Autodesk Inventor part; units mm, degrees
ref_plane "Work Plane3" through (0, 0, 2) normal (0, 0, 1) x (1, 0, 0)
ref_plane "Work Plane4" through (0, 0, -21) normal (0, 0, 1) x (1, 0, 0)
ref_plane "YZ Plane" through (0, 0, 0) normal (1, 0, 0) x (0, 1, 0)
sketch "Sketch1" plane through (0, 0, 0) normal (0, 1, 0) x (-1, 0, 0)
  line L0 (0, 0) -> (21, 0)
  circle A0 centre (5.5, 3.75) radius 1.5
  line L1 (29, 8) -> (-8, 8)
  line L2 (10.5, 8) -> (10.5, 0) construction
  line L3 (0, -21) -> (-8, -21)
  line L4 (29, 2) -> (72.5, 2)
  line L5 (72.5, 2) -> (72.5, 8)
  line L6 (72.5, 8) -> (29, 8)
  line L7 (29, 8) -> (29, 2)
  line L8 (21, 0) -> (21, 8)
  line L9 (0, 0) -> (0, 8)
  circle A1 centre (15.5, 3.75) radius 2.5
  line L10 (0, 0) -> (0, -21)
  line L11 (-8, -21) -> (-8, 8)
  line L12 (21, -21) -> (21, 0)
  line L13 (29, -21) -> (29, 2)
  line L14 (21, -21) -> (29, -21)
  circle A2 centre (-4, -10.5) radius 2.5
  circle A3 centre (25, -10.5) radius 1.5
  point P0 (29, 8)
  point P1 (21, 8)
  point P2 (-4, -21)
  dimension "d1" = 21
  dimension "d15" = 3.75
  dimension "d16" = 5
  dimension "d51" = 6
  dimension "d148" = 5
  dimension "d149" = 3.75
  dimension "d150" = 5
  dimension "d151" = 3
  dimension "d152" = 8
  dimension "d154" = 37
  dimension "d155" = 10.5
  dimension "d158" = 21
  dimension "d160" = 8
  dimension "d162" = 8
  dimension "d164" = 21
  dimension "d165" = 29
  dimension "d166" = 29
  dimension "d169" = 62
  dimension "d170" = 4
  dimension "d171" = 5
  dimension "d172" = 10.5
  dimension "d173" = 4
  dimension "d174" = 3
  dimension "d175" = 10.5
extrude "Extrusion1" add sketch "Sketch1" along normal mid plane 14 contours L9 L1 L8 L0 | L10 L3 L11 L1 L9 | L8 L1 L7 L13 L14 L12
extrude "Extrusion2" add sketch "Sketch1" along normal mid plane 25 contours L6 L5 L4 L7
fillet "Fillet4" radius 8 3 edges at (-72.5, 12.5, 5) (-72.5, -12.5, 5) (8, 0, 8)
ref_plane "Work Plane3" through (0, 0, 2) normal (0, 0, 1) x (1, 0, 0)
sketch "Sketch5" plane through (0, 0, 2) normal (0, 0, 1) x (1, 0, 0)
  line L0 (-29, -7) -> (-29, 7)
  circle A0 centre (-60.5, 0) radius 7.5
  line L1 (-21, -7) -> (0, -7)
  line L2 (-29, 12.5) -> (-64.5, 12.5)
  point P0 (0, 0)
  point P1 (-12.116, -8.0773)
  point P2 (-29, 0)
  point P3 (-10.5, -7)
  dimension "d195" = 15
  dimension "d196" = 50
  dimension "d197" = 12.5
extrude "Extrusion6" cut sketch "Sketch5" along normal blind 6
fillet "Fillet12" radius 2 13 edges at (-72.5, 0, 8) (-46.75, 12.5, 8) (-70.1569, -10.1569, 2) (-72.5, 0, 2) (-70.1569, 10.1569, 2) (-46.75, 12.5, 2) (-46.75, -12.5, 2) (5.6569, 7, 5.6569) (8, 7, -10.5) (-14.5, 7, 8) (5.6569, -7, 5.6569) (8, -7, -10.5) (-14.5, -7, 8)
ref_plane "Work Plane4" through (0, 0, -21) normal (0, 0, 1) x (1, 0, 0)
sketch "Sketch6" plane through (0, 0, -21) normal (0, 0, 1) x (1, 0, 0)
  line L0 (6, -4) -> (2, -4)
  line L1 (2, -4) -> (2, 4)
  line L2 (2, 4) -> (6, 4)
  line L3 (6, 4) -> (6, -4)
  line L4 (6, -4) -> (2, 4) construction
  line L5 (2, -4) -> (6, 4) construction
  line L6 (0, -7) -> (0, 7)
  line L7 (-23.1, -3.9) -> (-26.9, -3.9)
  line L8 (-26.9, -3.9) -> (-26.9, 3.9)
  line L9 (-26.9, 3.9) -> (-23.1, 3.9)
  line L10 (-23.1, 3.9) -> (-23.1, -3.9)
  line L11 (-23.1, -3.9) -> (-26.9, 3.9) construction
  line L12 (-26.9, -3.9) -> (-23.1, 3.9) construction
  line L13 (-21, -7) -> (-21, 7)
  point P0 (0, 0)
  point P1 (4, 0)
  point P2 (0, 0)
  point P3 (0, 0)
  point P4 (-25, 0)
  point P5 (-21, 0)
  dimension "d183" = 8
  dimension "d184" = 4
  dimension "d185" = 4
  dimension "d186" = 0
  dimension "d187" = 7.8
  dimension "d188" = 3.8
  dimension "d189" = 4
  dimension "d190" = 0
extrude "Extrusion12" add sketch "Sketch6" against normal blind 4 contours L7 L8 L9 L10
extrude "Extrusion13" cut sketch "Sketch6" along normal blind 4 contours L0 L1 L2 L3
equation "\"HoleDiameter\" = 3"
equation "\"InsertDiameter\" = 5"
equation "\"CoxaWidth\" = 25"
equation "\"SlotWidth1\" = 4"
equation "\"SlotLength1\" = 8"
equation "\"SlotHeight1\" = 4"
properties part number "ServoMount"
Verification items for the finished model (mm, model axes). A direction names the side the tool comes from. Round coordinates to 2 decimals unless told otherwise and drop trailing zeros. Order: outer loops, then holes, each group sorted by start corner. A loop starts at its lowest first (then second) coordinate and runs counter-clockwise, first axis right, second up. Notation, with made-up numbers: (-31.5, 58) -> (-20.5, 58) arc R23 cw to (-20.5, 89) -> close; hole circle Ø9 at (-15, 24.25). An arc over 180 degrees is marked (long way). Put each result on its own line as item: value. Start each with the question number.
(1) Section check A-A (y = 0). State how many separate pieces and enclosed holes the cut face has, then the cut area to 3 significant figures.
(2) Section check B-B (x = -5.5). Enter the section's corners in (y, z).
(3) Depth check by flat-ended pin: pin 1 Ø1.8 at (y, z) = (10, 5) entering from +X; pin 2 Ø6 at (x, z) = (-15.5, 3.75) entering from +Y; pin 3 Ø4 at (x, z) = (-25, -10.5) entering from -Y; pin 4 Ø2.5 at (x, z) = (-5.5, 3.75) entering from +Y. Enter the tip coordinate at first touch or a pass-through.
(4) Material ranges on line 1 along Z through (x, y) = (-5.5, 0.75); line 2 along X through (y, z) = (-2, -11); line 3 along X through (y, z) = (6.75, -11.5), recorded low to high.
(5) Section check D-D (x = -60.5). Enter the section's corners in (y, z), then the cut area to 3 significant figures.
(6) Section check C-C (z = -1). Enter the section's corners in (x, y), then the cut area to 3 significant figures.
(7) Draft check along Z on faces 4 (the face through (4, 0, -17)), 5 (the face through (-13.002, -0.098, 3.64)), 6 (the face through (-47, 12.5, 5)). Enter one of: +Z half, -Z half, draft (parallel to the pull), parting line (faces both ways), or undercut.
(8) Tool access check on faces 1 (the face through (6, 0, -19)), 2 (the face through (-21, 0, -11)), 3 (the face through (7.43, -6.4, -16.56)). Record the directions out of +Z, -Z, +X, -X, +Y, -Y that give a thin tool (end or side, any length) a straight path to the whole face; none if there is none.
Completed:
1. separate pieces: 2
1. enclosed holes: 4
1. area: 733 mm2
2. outline: (-7, 0) -> (7, 0) -> (7, 2.25) -> (-7, 2.25) -> close; (-7, 5.25) -> (7, 5.25) -> (7, 6) arc R2 ccw to (5, 8) -> (-5, 8) arc R2 ccw to (-7, 6) -> close
3. pin 1: stops at x = -29
3. pin 2: stops at y = 7
3. pin 3: stops at y = -7
3. pin 4: passes through
4. line 1: z = 0 to 2.25, 5.25 to 8
4. line 2: x = -29 to -26.41, -23.59 to -21, 0 to 1.55, 6.45 to 8
4. line 3: x = -29 to -26.12, -23.88 to -21, 0 to 1.71, 6.29 to 7.01
5. outline: (-12.5, 4) arc R2 ccw to (-10.5, 2) -> (-7.5, 2) -> (-7.5, 8) -> (-10.5, 8) arc R2 ccw to (-12.5, 6) -> close; (7.5, 2) -> (10.5, 2) arc R2 ccw to (12.5, 4) -> (12.5, 6) arc R2 ccw to (10.5, 8) -> (7.5, 8) -> close
5. area: 56.6 mm2
6. outline: (-29, -7) -> (-21, -7) -> (-21, 7) -> (-29, 7) -> close; (0, -7) -> (6, -7) arc R2 ccw to (8, -5) -> (8, 5) arc R2 ccw to (6, 7) -> (0, 7) -> close
6. area: 222 mm2
7. face 4: -Z half
7. face 5: undercut
7. face 6: draft
8. face 1: -Z
8. face 2: -Z, +Y, -Y
8. face 3: -Z, +X, -Y
